Source: CAD feature listing. Evaluate the final solid. Frame: model axes, mm. Give positions to 0.01 mm unless a question says otherwise; leave off trailing zeros. Order: outer loops, then holes, each group sorted by start corner. A loop starts at its lowest first (then second) coordinate and runs counter-clockwise, first axis right, second up. Notation, with made-up numbers: M 24.25,-22 L 36.25,-22 A31 cw 36.25,13 Z; hole C 89,-23.75 d9. An arc over 180 degrees is marked long. Return JSON: item names as keys, results as strings.
from build123d import *

# Parameters (mm, degrees)
SKETCH_1_W            = 275
SKETCH_1_H            = 204
SKETCH_1_W_2          = 8
SKETCH_1_H_2          = 44
EXTRUDE_1_DEPTH       = 3
SKETCH_2_R            = 2
SKETCH_2_R_2          = 57.5
SKETCH_2_R_3          = 2.25
CUT_EXTRUDE_1_DEPTH   = 3
SKETCH_3_W            = 119.5
SKETCH_3_H            = 119.5
CUT_EXTRUDE_2_DEPTH   = 2
FILLET_1_R            = 2
SKETCH_5_W            = 215
SKETCH_5_H            = 10
SKETCH_5_W_2          = 97.5
SKETCH_5_W_3          = 102.5
CUT_EXTRUDE_1_2_DEPTH = 3
FILLET_2_R            = 5
FILLET_3_R            = 2


with BuildPart() as part:
    # 스케치1 → 보스-돌출1 (new body)
    with BuildSketch(Plane.XY):
        Rectangle(SKETCH_1_W, SKETCH_1_H)
        Polygon((137.5, 58), (137.5, -70), (157.5, -70), (157.5, 58), (145.5, 58), align=None)
        with Locations((141.5, 80)):
            Rectangle(SKETCH_1_W_2, SKETCH_1_H_2)
    extrude(amount=EXTRUDE_1_DEPTH)

    # 스케치2 → Cut-Extrude 1 (cut)
    with BuildSketch(Plane.XY.offset(3)):
        with Locations((-126.9, 95)):
            Circle(SKETCH_2_R)
        with Locations((121.5, 95)):
            Circle(SKETCH_2_R)
        with Locations((-126.9, -95)):
            Circle(SKETCH_2_R)
        with Locations((121.5, -95)):
            Circle(SKETCH_2_R)
        with Locations((-52.5, 0)):
            Circle(SKETCH_2_R_2)
        with Locations((-105, 52.5)):
            Circle(SKETCH_2_R_3)
        with Locations((0, 52.5)):
            Circle(SKETCH_2_R_3)
        with Locations((0, -52.5)):
            Circle(SKETCH_2_R_3)
        with Locations((-105, -52.5)):
            Circle(SKETCH_2_R_3)
    extrude(amount=-CUT_EXTRUDE_1_DEPTH, mode=Mode.SUBTRACT)

    # 스케치3 → 컷-돌출2 (cut)
    with BuildSketch(Plane(origin=(0, 0, 0), x_dir=(-1, 0, 0), z_dir=(0, 0, -1))):
        with Locations((52.5, 0)):
            Rectangle(SKETCH_3_W, SKETCH_3_H)
    extrude(amount=-CUT_EXTRUDE_2_DEPTH, mode=Mode.SUBTRACT)

    # 필렛1
    fillet_1_edges = [part.edges().sort_by_distance(p)[0] for p in [
        (7.25, 59.75, 1),
        (-112.25, 59.75, 1),
        (-112.25, -59.75, 1),
        (7.25, -59.75, 1),
    ]]
    fillet(fillet_1_edges, radius=FILLET_1_R)

    # 스케치5 → Cut-Extrude 1 2 (cut)
    with BuildSketch(Plane.XY.offset(3)):
        with Locations((0, -80)):
            Rectangle(SKETCH_5_W, SKETCH_5_H)
        with Locations((73.75, -60)):
            Rectangle(SKETCH_5_W_2, SKETCH_5_H)
        with Locations((76.25, -40)):
            Rectangle(SKETCH_5_W_3, SKETCH_5_H)
        with Locations((76.25, -20)):
            Rectangle(SKETCH_5_W_3, SKETCH_5_H)
        with Locations((76.25, 0)):
            Rectangle(SKETCH_5_W_3, SKETCH_5_H)
        with Locations((76.25, 20)):
            Rectangle(SKETCH_5_W_3, SKETCH_5_H)
        with Locations((76.25, 40)):
            Rectangle(SKETCH_5_W_3, SKETCH_5_H)
        with Locations((73.75, 60)):
            Rectangle(SKETCH_5_W_2, SKETCH_5_H)
        with Locations((0, 80)):
            Rectangle(SKETCH_5_W, SKETCH_5_H)
    extrude(amount=-CUT_EXTRUDE_1_2_DEPTH, mode=Mode.SUBTRACT)

    # 필렛2
    fillet_2_edges = [part.edges().sort_by_distance(p)[0] for p in [
        (107.5, -85, 1.5),
        (122.5, -65, 1.5),
        (127.5, -45, 1.5),
        (127.5, -25, 1.5),
        (127.5, -5, 1.5),
        (127.5, 15, 1.5),
        (127.5, 35, 1.5),
        (122.5, 55, 1.5),
        (107.5, 75, 1.5),
        (25, 65, 1.5),
        (25, 45, 1.5),
        (25, 25, 1.5),
        (25, 5, 1.5),
        (25, -15, 1.5),
        (25, -35, 1.5),
        (25, -55, 1.5),
        (-107.5, -75, 1.5),
        (25, -65, 1.5),
        (25, -45, 1.5),
        (25, -25, 1.5),
        (25, -5, 1.5),
        (25, 15, 1.5),
        (25, 35, 1.5),
        (25, 55, 1.5),
        (-107.5, -85, 1.5),
        (127.5, 5, 1.5),
        (127.5, -15, 1.5),
        (127.5, -35, 1.5),
        (122.5, -55, 1.5),
        (107.5, -75, 1.5),
        (127.5, 25, 1.5),
        (122.5, 65, 1.5),
        (127.5, 45, 1.5),
        (107.5, 85, 1.5),
        (-107.5, 75, 1.5),
        (-107.5, 85, 1.5),
    ]]
    fillet(fillet_2_edges, radius=FILLET_2_R - 0.0001)  # a hair under: the kernel refuses the full size

    # 필렛3
    fillet_3_edges = [part.edges().sort_by_distance(p)[0] for p in [
        (157.5, 58, 1.5),
        (157.5, -70, 1.5),
        (137.5, -70, 1.5),
        (137.5, -102, 1.5),
        (-137.5, -102, 1.5),
        (-137.5, 102, 1.5),
        (145.5, 102, 1.5),
        (145.5, 58, 1.5),
    ]]
    fillet(fillet_3_edges, radius=FILLET_3_R)


solid = part.part
1. Section query D-D (y = 70.5). Return loops of the section in (x, z), then the cut area to 3 significant figures.
Evaluation:
{"outline": "M -137.5,0 L 145.5,0 L 145.5,3 L -137.5,3 Z", "area": "849 mm^2"}
2. Section query A-A (x = -52.5). Return loops of the section in (y, z), then the cut area to 3 significant figures.
Evaluation:
{"outline": "M -102,0 L -85,0 L -85,3 L -102,3 Z; M -75,0 L -59.75,0 L -59.75,2 L -57.5,2 L -57.5,3 L -75,3 Z; M 57.5,2 L 59.75,2 L 59.75,0 L 75,0 L 75,3 L 57.5,3 Z; M 85,0 L 102,0 L 102,3 L 85,3 Z", "area": "198 mm^2"}
3. Ray query, probe 1 along Y at (x, z) = (-14, 0.6); probe 2 along Y at (x, z) = (-126.9, 1.6); probe 3 along Y at (x, z) = (-52.5, 2.6). Return the intervals inside material, ascending.
Evaluation:
{"probe 1": "y = -102 to -85, -75 to -59.75, 59.75 to 75, 85 to 102", "probe 2": "y = -102 to -97, -93 to 93, 97 to 102", "probe 3": "y = -102 to -85, -75 to -57.5, 57.5 to 75, 85 to 102"}
4. Section query C-C (x = 82). State how many separate pieces and enclosed holes the cut face has, then the cut area to 3 significant figures.
Evaluation:
{"separate pieces": "10", "enclosed holes": "0", "area": "342 mm^2"}
5. Draft query along Y for faces 1 (the face through (8, 1, 3)), 2 (the face through (5.3, 0.3, 2)). Return one class per face: pulls with the +Y half, pulls with the -Y half, needs draft (parallel to the pull), parting line crosses it, or undercut.
Evaluation:
{"face 1": "needs draft", "face 2": "undercut"}
6. Section query B-B (y = 28). Return loops of the section in (x, z), then the cut area to 3 significant figures.
Evaluation:
{"outline": "M -137.5,0 L -112.25,0 L -112.25,2 L -102.72,2 L -102.72,3 L -137.5,3 Z; M -2.28,2 L 7.25,2 L 7.25,0 L 157.5,0 L 157.5,3 L -2.28,3 Z", "area": "546 mm^2"}
